Geometry check sheet. Reference: drawing and pictorial views, mm from the part's lowest x, y, z. Round coordinates to 2 decimals unless told otherwise and drop trailing zeros. Order: outer loops, then holes, each group sorted by start corner. A loop starts at its lowest first (then second) coordinate and runs counter-clockwise, first axis right, second up.
(1) Sectioned sample at D-D, the plane y = 6.5. Enter the section's corners in (x, z), and give its area (3 significant figures).
(2) Mould release check, pull along Z, two halves, no side actions. Record for the marked faces 1, 2, 3 and 4: released by +Z, released by -Z, zero draft, split by the parting line, or undercut.
(3) Depth check by flat-ended pin: pin 1 (7 mm diameter, centred on x = 28.5, z = 11, fed in from +Y); pin 2 (3.5 mm diameter, centred on x = 7.5, z = 11, fed in from +Y); pin 3 (14.5 mm diameter, centred on x = 8.5, z = 20, fed in from +Y); pin 4 (5 mm diameter, centred on x = 30, z = 22, fed in from +Y). Enter the tip coordinate at first touch or a pass-through.
(4) Sectioned sample at A-A, the plane z = 11. Enter the section's corners in (x, y), and give its area (3 significant figures).
(5) Thickness scan on probe 1 along X at (y, z) = (0.55, 11); probe 2 along Z at (x, y) = (7.5, 0.35); probe 3 along Z at (x, y) = (7.5, 1.5). Record the ranges inside material, lowest first.
(6) Sectioned sample at C-C, the plane z = 42.5. Enter the section's corners in (x, y).
(7) Sectioned sample at B-B, the plane x = 7.5. Enter the section's corners in (y, z), and give its area (3 significant figures).
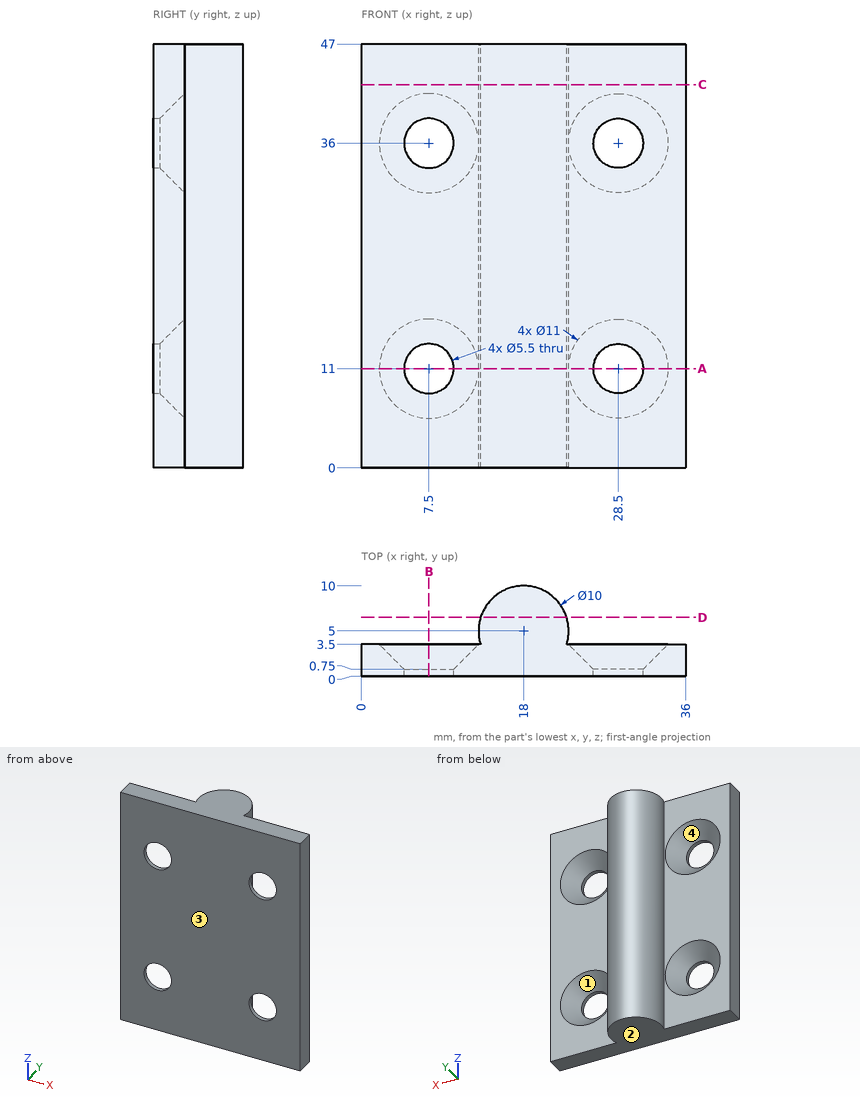
Derived:
1. outline: (13.23, 0) - (22.77, 0) - (22.77, 47) - (13.23, 47) - close
1. area: 448 mm2
2. face 1: undercut
2. face 2: released by -Z
2. face 3: zero draft
2. face 4: undercut
3. pin 1: stops at y = 1.5
3. pin 2: passes through
3. pin 3: stops at y = 9.47
3. pin 4: stops at y = 3.5
4. outline: (0, 0) - (4.75, 0) - (4.75, 0.75) - (2, 3.5) - (0, 3.5) - close; (10.25, 0) - (25.75, 0) - (25.75, 0.75) - (23, 3.5) - (22.77, 3.5) arc R5 ccw (long way) to (13.23, 3.5) - (13, 3.5) - (10.25, 0.75) - close; (31.25, 0) - (36, 0) - (36, 3.5) - (34, 3.5) - (31.25, 0.75) - close
4. area: 126 mm2
5. probe 1: x = 0 to 4.75, 10.25 to 25.75, 31.25 to 36
5. probe 2: z = 0 to 8.25, 13.75 to 33.25, 38.75 to 47
5. probe 3: z = 0 to 7.5, 14.5 to 32.5, 39.5 to 47
6. outline: (0, 0) - (36, 0) - (36, 3.5) - (22.77, 3.5) arc R5 ccw (long way) to (13.23, 3.5) - (0, 3.5) - close
7. outline: (0, 0) - (3.5, 0) - (3.5, 5.5) - (0.75, 8.25) - (0, 8.25) - close; (0, 13.75) - (0.75, 13.75) - (3.5, 16.5) - (3.5, 30.5) - (0.75, 33.25) - (0, 33.25) - close; (0, 38.75) - (0.75, 38.75) - (3.5, 41.5) - (3.5, 47) - (0, 47) - close
7. area: 111 mm2
